Verification items for the finished model (mm, model axes). A direction names the side the tool comes from. Coordinates: 2 decimals unless noted, no trailing zeros. Loops run counter-clockwise (first coordinate to the right, second up) from the corner with the lowest first, then second, coordinate; pieces in that order, holes last.
Q1. Access from +Z, -Z, +X, -X, +Y, -Y to the whole of each face (thin tool, end or side, straight path). Record for faces 4 (the face through (14, 98.274, 2)), 5 (the face through (-37.746, -1, 2)).
Q2. Material ranges on probe 1 along Y at (x, z) = (1, 0.45); probe 2 along X at (y, z) = (91.5, 2.15), recorded low to high.
Q3. Go/stop test with a flat-tipped pin: P1, Ø6, axis at x = 17, y = 4.5, coming from the -Z side. Record where the tip stops, or that it passes through.
Q4. Sectioned sample at C-C (z = 3.1). Enter the section's corners in (x, y), then the cut area to 3 significant figures.
Q5. Sectioned sample at A-A (y = -30). Enter the section's corners in (x, z), then the cut area to 3 significant figures.
Q6. Sectioned sample at B-B (x = 34.5). Enter the section's corners in (y, z).
Q7. Mould release check, pull along X, two halves, no side actions. Record for faces 1 (the face through (66.254, -4, 2)), 2 (the face through (-1, -2, 5)), 3 (the face through (14, -103.274, 2)): +X half, -X half, draft (parallel to the pull), parting line (faces both ways), or undercut.
```python
from build123d import *

# Parameters (mm, degrees)
F0_W     = 100
F0_H     = 5
F1_DEPTH = 5


with BuildPart() as f1:
    # F0 (on Top) → F1 (new body)
    with BuildSketch(Plane.XY):
        Polygon((-35.745753, 98.273505), (-35.745753, 103.273505), (-37.745753, 103.273505), (-37.745753, -108.273505), (-35.745753, -108.273505), (-35.745753, -103.273505), (-35.745753, -5), (-35.745753, 0), align=None)
        with Locations((14.254247, -105.773505)):
            Rectangle(F0_W, F0_H)
        with Locations((14.254247, -2.5)):
            Rectangle(F0_W, F0_H)
        with Locations((14.254247, 100.773505)):
            Rectangle(F0_W, F0_H)
        Polygon((66.254247, 103.273505), (64.254247, 103.273505), (64.254247, 98.273505), (64.254247, 0), (64.254247, -5), (64.254247, -103.273505), (64.254247, -108.273505), (66.254247, -108.273505), align=None)
    extrude(amount=F1_DEPTH)


solid = f1.part
```
Geometry check:
1. face 4: +Z, -Z
1. face 5: +Z, -Z, -X, +Y, -Y
2. probe 1: y = -108.27 to -103.27, -5 to 0, 98.27 to 103.27
2. probe 2: x = -37.75 to -35.75, 64.25 to 66.25
3. P1: passes through
4. outline: (-37.75, -108.27) - (66.25, -108.27) - (66.25, 103.27) - (-37.75, 103.27) - close; hole (-35.75, -103.27) - (64.25, -103.27) - (64.25, -5) - (-35.75, -5) - close; hole (-35.75, 0) - (64.25, 0) - (64.25, 98.27) - (-35.75, 98.27) - close
4. area: 2,350 mm2
5. outline: (-37.75, 0) - (-35.75, 0) - (-35.75, 5) - (-37.75, 5) - close; (64.25, 0) - (66.25, 0) - (66.25, 5) - (64.25, 5) - close
5. area: 20.0 mm2
6. outline: (-108.27, 0) - (-103.27, 0) - (-103.27, 5) - (-108.27, 5) - close; (-5, 0) - (0, 0) - (0, 5) - (-5, 5) - close; (98.27, 0) - (103.27, 0) - (103.27, 5) - (98.27, 5) - close
7. face 1: +X half
7. face 2: draft
7. face 3: undercut
